Check sheet for the modelled part. Datum: model origin and axes. Units: mm. A direction names the side the tool comes from. Round coordinates to 2 decimals unless told otherwise and drop trailing zeros. Write each loop counter-clockwise with the first axis right and the second up, starting at its lowest first coordinate (ties: lowest second). Pieces come first, ordered by that corner, then holes.
Item 1: Section check B-B, the plane y = -11. Record the cut outline in (x, z).
Item 2: Depth check by flat-ended pin: pin 1 (1.5 mm diameter, centred on x = -1, z = 11.5, fed in from -Y); pin 2 (2 mm diameter, centred on y = -22, z = 16, fed in from -X); pin 3 (5 mm diameter, centred on x = 15.5, y = -27.5, fed in from -Z). Enter the tip coordinate at first touch or a pass-through.
Item 3: Release check for a two-part mould opening along Z. For faces 1 (the cylindrical face through (-0.733, -16.041, -12.09)), 2 (the flat face through (0, -25.4, 0)) record: pulls with the +Z half, pulls with the -Z half, needs draft (parallel to the pull), parting line crosses it, or undercut.
Item 4: Section check D-D, the plane y = -17.5. Record the cut outline in (x, z), plus the area to 3 significant figures.
Item 5: Set-up check for faces 3 (the flat face through (-12.7, -13, 0)), 4 (the flat face through (0, 0, 3)): record each of +Z, -Z, +X, -X, +Y, -Y from which the full face is reachable in a straight line by a thin tool's end or side.
Item 6: Material ranges on line 1 along Z through (x, y) = (-9.5, -23); line 2 along Y through (x, z) = (0, -17); line 3 along X through (y, z) = (-23, -1.5), recorded low to high.
Item 7: Section check A-A, the plane x = 0. Record the cut outline in (y, z) (3 decimals).
Item 8: Section check C-C, the plane z = -5. Record the cut outline in (x, y) (1 decimal), plus the area to 3 significant figures.
from build123d import *

# Parameters (mm, degrees)
F0_W     = 12.7
F0_H     = 4.7625
F1_DEPTH = 25.4
F2_D     = 3.175
F2_DEPTH = 21.591
F5_D     = 3.175


with BuildPart() as f4:
    # F3 (on Top) → F4 (revolve)
    with BuildSketch(Plane.XY):
        with BuildLine():
            Line((0, -36.2225826497), (0, 0))
            Line((0, 0), (-15.875, 0))
            ThreePointArc((-15.875, 0), (-19.7742959345, -23.2989152245), (0, -36.2225826497))
        make_face()
    revolve(axis=Axis((0, -18.1112913248, 0), (0, -1, 0)))

    # F0 (on Front) → F1 (cut)
    with BuildSketch(Plane.XZ):
        with Locations((6.35, 0)):
            Rectangle(F0_W, F0_H)
        with Locations((-6.35, 0)):
            Rectangle(F0_W, F0_H)
    extrude(amount=F1_DEPTH, mode=Mode.SUBTRACT)

    # F2 (through all, one way)
    with BuildSketch(Plane(origin=(0, 0, 0), x_dir=(1, 0, 0), z_dir=(0, 0, -1))):
        with Locations((0, 14.6325826497)):
            Circle(F2_D / 2)
    extrude(amount=-F2_DEPTH, mode=Mode.SUBTRACT)

    # F5 (through all)
    with Locations(Plane.XY):
        with Locations((0, -14.6325826497)):
            Hole(F5_D / 2)


solid = f4.part
Values found:
1. outline: circle Ø42.56 at (0, 0); hole (-12.7, -2.38) - (12.7, -2.38) - (12.7, 2.38) - (-12.7, 2.38) - close
2. pin 1: stops at y = -33.33
2. pin 2: stops at x = -13.79
2. pin 3: stops at z = -12.44
3. face 1: needs draft
3. face 2: undercut
4. outline: circle Ø42.8 at (0, 0); hole (-12.7, -2.38) - (12.7, -2.38) - (12.7, 2.38) - (-12.7, 2.38) - close
4. area: 1,320 mm2
5. face 3: +Y
5. face 4: +Z, -Z, +X, -X, +Y
6. line 1: z = -17.49 to -2.38, 2.38 to 17.49
6. line 2: y = -27.94 to -16.22, -13.05 to -1.32
6. line 3: x = -19.85 to -12.7, 12.7 to 19.85
7. outline: (-25.4, -2.381) - (-25.4, 2.381) - (-16.22, 2.381) - (-16.22, 21.532) arc R21.59 ccw to (-16.22, -21.532) - (-16.22, -2.381) - close; (-13.045, -21.532) arc R21.59 ccw to (0, -15.875) - (0, -2.381) - (-13.045, -2.381) - close; (-13.045, 2.381) - (0, 2.381) - (0, 15.875) arc R21.59 ccw to (-13.045, 21.532) - close
8. outline: (-15.1, 0) arc R21 ccw (long way) to (15.1, 0) - close; hole circle Ø3.2 at (0, -14.6)
8. area: 1,250 mm2
